Can you work these out from the drawing? Everything is in mm from the part's minimum corner. Give positions to 0.01 mm unless a question says otherwise; leave off trailing zeros. Write each loop counter-clockwise with the first axis right and the second up, starting at its lowest first coordinate (ties: lowest second). Pieces come first, ordered by that corner, then holes. Notation, with made-up numbers: (30, 15) - (43, 15) arc R26 ccw to (43, 43) - close; hole circle Ø4 at (72.5, 85). An arc over 180 degrees is marked (long way). Answer in a Markdown table with one row per item.
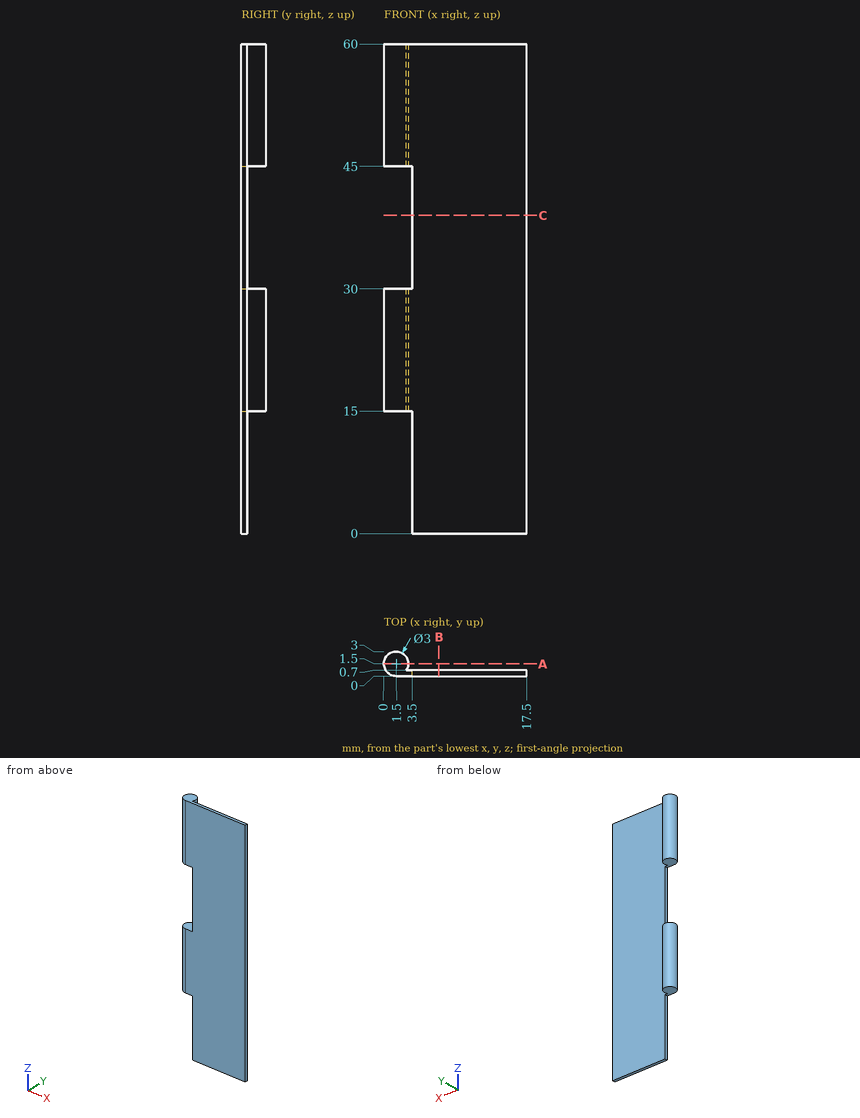
1) Imagine slicing it at C-C (z = 39). List the corners of the cut face in (x, y) for me.
Check values:
| item | result |
|---|---|
| outline | (3.5, 0) - (17.5, 0) - (17.5, 0.7) - (3.5, 0.7) - close |
2) Imagine slicing it at A-A (y = 1.5). List the corners of the cut face in (x, z) for me, then the cut area to 3 significant figures.
Check values:
| item | result |
|---|---|
| outline | (0, 15) - (3, 15) - (3, 30) - (0, 30) - close; (0, 45) - (3, 45) - (3, 60) - (0, 60) - close |
| area | 90.0 mm2 |
3) If I drill on line 1 (Z direction, x = 1, y = 2.05); line 2 (Y direction, x = 15, z = 12); line 3 (X direction, y = 2.75, z = 20.5), over which ranges is the centre line in solid material (lowest first)?
Check values:
| item | result |
|---|---|
| line 1 | z = 15 to 30, 45 to 60 |
| line 2 | y = 0 to 0.7 |
| line 3 | x = 0.67 to 2.33 |
4) Imagine slicing it at B-B (x = 6.75). List the corners of the cut face in (y, z) for me.
Check values:
| item | result |
|---|---|
| outline | (0, 0) - (0.7, 0) - (0.7, 60) - (0, 60) - close |
5) Will these pins go through, and if not, where does the flat tip stop? P1, Ø0.6, axis at y = 0, z = 34.5, coming from the -X side; P2, Ø1, axis at y = 2, z = 53.5, coming from the +X side; P3, Ø1, axis at x = 9.5, y = 2, coming from the -Z side.
Check values:
| item | result |
|---|---|
| P1 | stops at x = 3.5 |
| P2 | stops at x = 3 |
| P3 | passes through |
